Here's how the part is built. I have some questions about the finished solid (model axes, mm). Coordinates: 2 decimals unless noted, no trailing zeros. Order: outer loops, then holes, each group sorted by start corner. A loop starts at its lowest first (then second) coordinate and runs counter-clockwise, first axis right, second up. Notation, with made-up numbers: (52.5, 4.5) - (66.5, 4.5) arc R22 ccw to (66.5, 21.5) - close; hole circle Ø7 at (10, -39.75). An arc over 180 degrees is marked (long way). Answer as CSV lines item,"result". Start each with the question number.
Q1. Suppose I cut it at C-C (z = -32). Please give me the cut outline in (x, y) (3 decimals).
Q2. Suppose I cut it at A-A (y = 0). Please give me the cut outline in (x, z) (3 decimals), then the cut area to 3 significant figures.
Q3. Suppose I cut it at D-D (x = 2.5). Count the separate pieces of the cut face and the enclosed holes in it, then the cut area to 3 significant figures.
Q4. Thinking about a two-plate mould opening in Z: for faces 1 (the face through (1.565, -8.899, 20.685)), 2 (the face through (1.57, 14.5, -46.03)), 3 (the face through (0, 1, -21)), which applies, released by +Z, released by -Z, zero draft, split by the parting line, or undercut?
Q5. I need wall thicknesses on line 1 (Y direction, x = 2.2, z = -7.5); line 2 (Y direction, x = 1.3, z = 33); line 3 (Z direction, x = 0.4, y = 9.5). Which ranges of each line are inside material? Lowest first, please.
from build123d import *

# Parameters (mm, degrees)
SKETCH1_R           = 48.26
SKETCH1_R_2         = 2.15265
SKETCH1_R_3         = 3.5
SKETCH1_R_4         = 17.5
BOSS_EXTRUDE1_DEPTH = 3.175


with BuildPart() as part:
    # Sketch1 → Boss-Extrude1 (new body)
    with BuildSketch(Plane(origin=(0, 0, 0), x_dir=(0, 0, -1), z_dir=(1, 0, 0))):
        Circle(SKETCH1_R)
        with Locations((0, 45.085)):
            Circle(SKETCH1_R_2, mode=Mode.SUBTRACT)
        with Locations((-24.023795501, -9.950801949)):
            Circle(SKETCH1_R_3, mode=Mode.SUBTRACT)
        with Locations((31.87990923, 31.87990923)):
            Circle(SKETCH1_R_2, mode=Mode.SUBTRACT)
        with Locations((45.085, 0)):
            Circle(SKETCH1_R_2, mode=Mode.SUBTRACT)
        with Locations((24.018239985, 9.948012748)):
            Circle(SKETCH1_R_3, mode=Mode.SUBTRACT)
        with Locations((-9.9503853, 24.023968076)):
            Circle(SKETCH1_R_3, mode=Mode.SUBTRACT)
        with Locations((31.87990923, -31.87990923)):
            Circle(SKETCH1_R_2, mode=Mode.SUBTRACT)
        with Locations((0, -45.085)):
            Circle(SKETCH1_R_2, mode=Mode.SUBTRACT)
        with Locations((-31.87990923, -31.87990923)):
            Circle(SKETCH1_R_2, mode=Mode.SUBTRACT)
        with Locations((-45.085, 0)):
            Circle(SKETCH1_R_2, mode=Mode.SUBTRACT)
        with Locations((-31.87990923, 31.87990923)):
            Circle(SKETCH1_R_2, mode=Mode.SUBTRACT)
        Circle(SKETCH1_R_4, mode=Mode.SUBTRACT)
        with Locations((9.950974523, -24.02421215)):
            Circle(SKETCH1_R_3, mode=Mode.SUBTRACT)
    extrude(amount=BOSS_EXTRUDE1_DEPTH)


solid = part.part
Here are the results:
1,outline,"(0, -36.125) - (3.175, -36.125) - (3.175, -34.029) - (0, -34.029) - close; (0, -29.731) - (3.175, -29.731) - (3.175, 29.731) - (0, 29.731) - close; (0, 34.029) - (3.175, 34.029) - (3.175, 36.125) - (0, 36.125) - close"
2,outline,"(0, -48.26) - (3.175, -48.26) - (3.175, -47.238) - (0, -47.238) - close; (0, -42.932) - (3.175, -42.932) - (3.175, -17.5) - (0, -17.5) - close; (0, 17.5) - (3.175, 17.5) - (3.175, 42.932) - (0, 42.932) - close; (0, 47.238) - (3.175, 47.238) - (3.175, 48.26) - (0, 48.26) - close"
2,area,"168 mm²"
3,separate pieces,"1"
3,enclosed holes,"13"
3,area,"6,080 mm²"
4,face 1,"undercut"
4,face 2,"split by the parting line"
4,face 3,"zero draft"
5,line 1,"y = -47.67 to -26.52, -21.53 to -15.81, 15.81 to 47.67"
5,line 2,"y = -35.21 to -33.72, -30.04 to 30.04, 33.72 to 35.21"
5,line 3,"z = -47.32 to -27.49, -20.55 to -14.7, 14.7 to 47.32"
